from build123d import *
from build123d.topology import SkipClean

# Parameters (mm, degrees)
SKETCH_1_R              = 2.5
SKETCH_1_W              = 47.2
SKETCH_1_H              = 66.2
SKETCH_1_R_2            = 1.5
SKETCH_1_W_2            = 89
SKETCH_1_H_2            = 34
EXTRUDE_1_DEPTH         = 10
FILLET_1_R              = 4
FILLET_4_R              = 6
FILLET_7_R              = 3
FILLET_8_R              = 3
SKETCH_2_R              = 2.5
SKETCH_2_R_2            = 1.5
CUT_EXTRUDE_1_DEPTH     = 258.430709124
SKETCH_3_R              = 2.5
CUT_EXTRUDE_2_DEPTH     = 30
SKETCH_4_R              = 1.5
CUT_EXTRUDE_3_DEPTH     = 263.774751451
FILLET_10_R             = 15
FILLET_11_R             = 3
FILLET_1_OF_MIRROR_1_R  = 4
FILLET_4_OF_MIRROR_1_R  = 6
FILLET_7_OF_MIRROR_1_R  = 3
FILLET_8_OF_MIRROR_1_R  = 3
FILLET_10_OF_MIRROR_1_R = 15
FILLET_11_OF_MIRROR_1_R = 3
SKETCH_5_R              = 2.5
EXTRUDE_2_DEPTH         = 10
SKETCH_6_R              = 2.5
CUT_EXTRUDE_4_DEPTH     = 10
EXTRUDE_3_DEPTH         = 10
SKETCH_8_R              = 2.5
CUT_EXTRUDE_5_DEPTH     = 10


with BuildPart() as part:
    # 草图1 → 凸台-拉伸1 (new body)
    with BuildSketch(Plane.XY):
        with BuildLine():
            Line((-46, -17), (-46, 17))
            Line((-46, 17), (0, 17))
            Line((0, 17), (0, 25))
            Line((0, 25), (-176.776511015, 25))
            ThreePointArc((-176.776511015, 25), (-184.605554742, 35.220778596), (-194.787701414, 43.1))
            Line((-194.787701414, 43.1), (-203.153806011, 41.1))
            Line((-203.153806011, 41.1), (-236.846193989, 41.1))
            Line((-236.846193989, 41.1), (-245.212298586, 43.1))
            ThreePointArc((-245.212298586, 43.1), (-249.567187761, 40.23743789), (-253.6, 36.936567247))
            Line((-253.6, 36.936567247), (-253.6, 25.2))
            ThreePointArc((-253.6, 25.2), (-252.623320065, 26.452201949), (-251.6, 27.666586345))
            Line((-251.6, 27.666586345), (-251.6, -27.666586345))
            ThreePointArc((-251.6, -27.666586345), (-252.623320065, -26.452201949), (-253.6, -25.2))
            Line((-253.6, -25.2), (-253.6, -36.936567247))
            ThreePointArc((-253.6, -36.936567247), (-249.567187761, -40.23743789), (-245.212298586, -43.1))
            Line((-245.212298586, -43.1), (-236.846193989, -41.1))
            Line((-236.846193989, -41.1), (-203.153806011, -41.1))
            Line((-203.153806011, -41.1), (-194.787701414, -43.1))
            ThreePointArc((-194.787701414, -43.1), (-184.605554742, -35.220778596), (-176.776511015, -25))
            Line((-176.776511015, -25), (0, -25))
            Line((0, -25), (0, -17))
            Line((0, -17), (-46, -17))
        make_face()
        with Locations((-51, 17)):
            Circle(SKETCH_1_R, mode=Mode.SUBTRACT)
        with Locations((-150, -19)):
            Circle(SKETCH_1_R, mode=Mode.SUBTRACT)
        with BuildLine():
            Line((-188.4, -27.666586345), (-188.4, 27.666586345))
            ThreePointArc((-188.4, 27.666586345), (-178, 0), (-188.4, -27.666586345))
        make_face(mode=Mode.SUBTRACT)
        with BuildLine():
            Line((-155, -17), (-173.050346114, -17))
            ThreePointArc((-173.050346114, -17), (-170.067345354, 0), (-173.050346114, 17))
            Line((-173.050346114, 17), (-155, 17))
            Line((-155, 17), (-155, -17))
        make_face(mode=Mode.SUBTRACT)
        with Locations((-51, -17)):
            Circle(SKETCH_1_R, mode=Mode.SUBTRACT)
        with Locations((-220, 0)):
            Rectangle(SKETCH_1_W, SKETCH_1_H, mode=Mode.SUBTRACT)
        with Locations((-150, 0)):
            Circle(SKETCH_1_R_2, mode=Mode.SUBTRACT)
        with Locations((-150, 19)):
            Circle(SKETCH_1_R, mode=Mode.SUBTRACT)
        with Locations((-100.5, 0)):
            Rectangle(SKETCH_1_W_2, SKETCH_1_H_2, mode=Mode.SUBTRACT)
        with Locations((-51, 0)):
            Circle(SKETCH_1_R_2, mode=Mode.SUBTRACT)
    extrude_1 = extrude(amount=EXTRUDE_1_DEPTH)

    # 圆角1
    fillet_1_edges = [part.edges().sort_by_distance(p)[0] for p in [
        (-196.4, 33.1, 5),
        (-243.6, 33.1, 5),
        (-243.6, -33.1, 5),
        (-196.4, -33.1, 5),
    ]]
    fillet(fillet_1_edges, radius=FILLET_1_R)

    # 圆角4
    fillet_4_edges = [part.edges().sort_by_distance(p)[0] for p in [
        (-155, -17, 5),
        (-155, 17, 5),
        (-145, 17, 5),
        (-145, -17, 5),
        (-56, -17, 5),
        (-56, 17, 5),
        (-46, -17, 5),
        (-46, 17, 5),
    ]]
    fillet(fillet_4_edges, radius=FILLET_4_R)

    # 圆角7
    # the kernel refuses this fillet: 3 mm, written as the material it adds along each edge
    with BuildSketch(Plane(origin=(-251.6, -27.666586345, 0), x_dir=(-0.6298143321188929, 0.7767457158283095, 0), z_dir=(0, 0, 1))) as fillet_7_piece_1:
        with BuildLine():
            CenterArc((6.002322024, -1.004638225), FILLET_7_R, 160.43479501, 70.528779366)
            Line((4.112879028, -3.334875372), (4.075090168, -3.381480115))
            Line((4.075090168, -3.381480115), (-0.03778886, -0.046604743))
            Line((-0.03778886, -0.046604743), (-0.002268242, 0.05995711))
            ThreePointArc((-0.002268242, 0.05995711), (1.58776952, 0.090022779), (3.119003381, 0.020092764))
            Line((3.119003381, 0.020092764), (3.175539041, 0))
        make_face()
    extrude(amount=10)
    with BuildSketch(Plane(origin=(-251.6, 27.666586345, 0), x_dir=(0, -1, 0), z_dir=(0, 0, 1))) as fillet_7_piece_2:
        with BuildLine():
            CenterArc((5.29501347, -3), FILLET_7_R, 90, 70.528779366)
            Line((2.466586345, -2), (2.410017803, -1.98))
            ThreePointArc((2.410017803, -1.98), (1.176595536, -1.069924808), (-0.039523695, -0.045142857))
            Line((-0.039523695, -0.045142857), (0, 0.06))
            Line((0, 0.06), (5.29501347, 0.06))
            Line((5.29501347, 0.06), (5.29501347, 0))
        make_face()
    extrude(amount=10)

    # 圆角8
    fillet_8_edges = [part.edges().sort_by_distance(p)[0] for p in [
        (-188.4, 27.666586345, 5),
        (-188.4, -27.666586345, 5),
    ]]
    fillet(fillet_8_edges, radius=FILLET_8_R)

    # 草图2 → 切除-拉伸1 (cut, symmetric)
    with BuildSketch(Plane(origin=(0, 0, 0), x_dir=(1, 0, 0), z_dir=(0, 1, 0))):
        with Locations(Location((-232.5, -5, 0), (0, 0, 270))):
            Circle(SKETCH_2_R)
        with Locations(Location((-207.5, -5, 0), (0, 0, 270))):
            Circle(SKETCH_2_R)
        with Locations(Location((-220, -5, 0), (0, 0, 270))):
            Circle(SKETCH_2_R_2)
    cut_extrude_1 = extrude(amount=CUT_EXTRUDE_1_DEPTH, both=True, mode=Mode.SUBTRACT)

    # 草图3 → 切除-拉伸2 (cut)
    with BuildSketch(Plane(origin=(-243.6, 0, 0), x_dir=(0, 0, -1), z_dir=(1, 0, 0))):
        with Locations((-5, 15)):
            Circle(SKETCH_3_R)
        with Locations((-5, -15)):
            Circle(SKETCH_3_R)
    cut_extrude_2 = extrude(amount=-CUT_EXTRUDE_2_DEPTH, mode=Mode.SUBTRACT)

    # 草图4 → 切除-拉伸3 (cut, through all)
    with BuildSketch(Plane(origin=(0, 25, 0), x_dir=(1, 0, 0), z_dir=(0, 1, 0))):
        with Locations((0, -5)):
            Circle(SKETCH_4_R)
    cut_extrude_3 = extrude(amount=-CUT_EXTRUDE_3_DEPTH, mode=Mode.SUBTRACT)

    # 圆角10
    fillet_10_edges = [part.edges().sort_by_distance(p)[0] for p in [
        (-176.776511015, -25, 5),
        (-176.776511015, 25, 5),
    ]]
    fillet(fillet_10_edges, radius=FILLET_10_R)

    # 圆角11
    fillet_11_edges = [part.edges().sort_by_distance(p)[0] for p in [
        (-173.050346114, 17, 5),
        (-173.050346114, -17, 5),
    ]]
    fillet(fillet_11_edges, radius=FILLET_11_R)

    # 镜向1: 凸台-拉伸1, 切除-拉伸1, 切除-拉伸2, 切除-拉伸3 across plane
    with SkipClean():  # the faces are left unmerged after this step: merging them gives an invalid solid
        add(extrude_1.mirror(Plane(origin=(0, 0, 10), x_dir=(0, 0, 1), z_dir=(1, 0, 0))))
        add(cut_extrude_1.mirror(Plane(origin=(0, 0, 10), x_dir=(0, 0, 1), z_dir=(1, 0, 0))), mode=Mode.SUBTRACT)
        add(cut_extrude_2.mirror(Plane(origin=(0, 0, 10), x_dir=(0, 0, 1), z_dir=(1, 0, 0))), mode=Mode.SUBTRACT)
        add(cut_extrude_3.mirror(Plane(origin=(0, 0, 10), x_dir=(0, 0, 1), z_dir=(1, 0, 0))), mode=Mode.SUBTRACT)

    # 圆角1 of 镜向1
    fillet_1_of_mirror_1_edges = [part.edges().sort_by_distance(p)[0] for p in [
        (196.4, 33.1, 5),
        (243.6, 33.1, 5),
        (243.6, -33.1, 5),
        (196.4, -33.1, 5),
    ]]
    fillet(fillet_1_of_mirror_1_edges, radius=FILLET_1_OF_MIRROR_1_R)

    # 圆角4 of 镜向1
    fillet_4_of_mirror_1_edges = [part.edges().sort_by_distance(p)[0] for p in [
        (155, -17, 5),
        (155, 17, 5),
        (145, 17, 5),
        (145, -17, 5),
        (56, -17, 5),
        (56, 17, 5),
        (46, -17, 5),
        (46, 17, 5),
    ]]
    fillet(fillet_4_of_mirror_1_edges, radius=FILLET_4_OF_MIRROR_1_R)

    # 圆角7 of 镜向1
    # the kernel refuses this fillet: 3 mm, written as the material it adds along each edge
    with BuildSketch(Plane(origin=(251.6, -27.666586345, 0), x_dir=(0, 1, 0), z_dir=(0, 0, 1))) as fillet_7_of_mirror_1_piece_1:
        with BuildLine():
            CenterArc((5.29501347, -3), FILLET_7_OF_MIRROR_1_R, 90, 70.528779366)
            Line((2.466586345, -2), (2.410017803, -1.98))
            ThreePointArc((2.410017803, -1.98), (1.176595536, -1.069924808), (-0.039523695, -0.045142857))
            Line((-0.039523695, -0.045142857), (0, 0.06))
            Line((0, 0.06), (5.29501347, 0.06))
            Line((5.29501347, 0.06), (5.29501347, 0))
        make_face()
    extrude(amount=10)
    with BuildSketch(Plane(origin=(251.6, 27.666586345, 0), x_dir=(0.6298143321188939, -0.7767457158283085, 0), z_dir=(0, 0, 1))) as fillet_7_of_mirror_1_piece_2:
        with BuildLine():
            CenterArc((6.002322024, -1.004638225), FILLET_7_OF_MIRROR_1_R, 160.43479501, 70.528779366)
            Line((4.112879028, -3.334875372), (4.075090168, -3.381480115))
            Line((4.075090168, -3.381480115), (-0.03778886, -0.046604743))
            Line((-0.03778886, -0.046604743), (-0.002268242, 0.05995711))
            ThreePointArc((-0.002268242, 0.05995711), (1.58776952, 0.090022779), (3.119003381, 0.020092764))
            Line((3.119003381, 0.020092764), (3.175539041, 0))
        make_face()
    extrude(amount=10)

    # 圆角8 of 镜向1
    fillet_8_of_mirror_1_edges = [part.edges().sort_by_distance(p)[0] for p in [
        (188.4, 27.666586345, 5),
        (188.4, -27.666586345, 5),
    ]]
    fillet(fillet_8_of_mirror_1_edges, radius=FILLET_8_OF_MIRROR_1_R)

    # 圆角10 of 镜向1
    fillet_10_of_mirror_1_edges = [part.edges().sort_by_distance(p)[0] for p in [
        (176.776511015, -25, 5),
        (176.776511015, 25, 5),
    ]]
    fillet(fillet_10_of_mirror_1_edges, radius=FILLET_10_OF_MIRROR_1_R)

    # 圆角11 of 镜向1
    fillet_11_of_mirror_1_edges = [part.edges().sort_by_distance(p)[0] for p in [
        (173.050346114, 17, 5),
        (173.050346114, -17, 5),
    ]]
    fillet(fillet_11_of_mirror_1_edges, radius=FILLET_11_OF_MIRROR_1_R)

    # 草图5 → 凸台-拉伸2 (add)
    with BuildSketch(Plane(origin=(0, 0, 0), x_dir=(-1, 0, 0), z_dir=(0, 0, -1))):
        with Locations((150, 19)):
            Circle(SKETCH_5_R)
        with Locations((150, -19)):
            Circle(SKETCH_5_R)
        with Locations((-150, -19)):
            Circle(SKETCH_5_R)
        with Locations((-150, 19)):
            Circle(SKETCH_5_R)
    extrude(amount=-EXTRUDE_2_DEPTH)

    # 草图6 → 切除-拉伸4 (cut)
    with BuildSketch(Plane(origin=(0, 0, 0), x_dir=(-1, 0, 0), z_dir=(0, 0, -1))):
        with Locations(Location((-150, 16, 0), (0, 0, 90))):
            Circle(SKETCH_6_R)
        with Locations(Location((-150, -16, 0), (0, 0, 270))):
            Circle(SKETCH_6_R)
        with Locations((48, -16)):
            Circle(SKETCH_6_R)
        with Locations((48, 16)):
            Circle(SKETCH_6_R)
    extrude(amount=-CUT_EXTRUDE_4_DEPTH, mode=Mode.SUBTRACT)

    # 草图7 → 凸台-拉伸3 (add)
    with BuildSketch(Plane(origin=(0, 0, 0), x_dir=(-1, 0, 0), z_dir=(0, 0, -1))):
        with BuildLine():
            ThreePointArc((48.887627564, 18.337117307), (45.628291755, 15.209430585), (50.112372436, 14.662882693))
            ThreePointArc((50.112372436, 14.662882693), (48.628291755, 16.209430585), (48.887627564, 18.337117307))
        make_face()
        with BuildLine():
            ThreePointArc((50.112372436, -14.662882693), (48.628291755, -16.209430585), (48.887627564, -18.337117307))
            ThreePointArc((48.887627564, -18.337117307), (45.628291755, -15.209430585), (50.112372436, -14.662882693))
        make_face()
    extrude(amount=-EXTRUDE_3_DEPTH)

    # 草图8 → 切除-拉伸5 (cut)
    with BuildSketch(Plane(origin=(0, 0, 0), x_dir=(-1, 0, 0), z_dir=(0, 0, -1))):
        with Locations(Location((-150, 16, 0), (0, 0, 90))):
            Circle(SKETCH_8_R)
        with Locations(Location((-150, -16, 0), (0, 0, 270))):
            Circle(SKETCH_8_R)
        with Locations(Location((150, -16, 0), (0, 0, 270))):
            Circle(SKETCH_8_R)
        with Locations(Location((150, 16, 0), (0, 0, 270))):
            Circle(SKETCH_8_R)
    extrude(amount=-CUT_EXTRUDE_5_DEPTH, mode=Mode.SUBTRACT)


solid = part.part
Model file for the job. Use its own axes, mm. A direction names the side the tool comes from. Give positions to 0.01 mm unless a question says otherwise; leave off trailing zeros. Loops run counter-clockwise (first coordinate to the right, second up) from the corner with the lowest first, then second, coordinate; pieces in that order, holes last. Notation, with made-up numbers: (63, 57) -> (67, 57) arc R22 cw to (67, 91) -> close; hole circle Ø2 at (-31, -2.75). An arc over 180 degrees is marked (long way). Use a Markdown table: item, result. Add a question column.
(1) Tool access for faces 1 (the flat face through (220, 41.1, 3)), 2 (the cylindrical face through (-187.242, -37.685, 4.93)), 3 (the flat face through (56, 0, 5)): list every direction of +Z, -Z, +X, -X, +Y, -Y with a clear straight run to the whole face (end or side of a thin tool).
(2) Drop flat-ended pins along their axis: pin 1 Ø5 at (x, z) = (11, 5) entering from +Y; pin 2 Ø3 at (x, z) = (216, 4.5) entering from +Y; pin 3 Ø3 at (x, z) = (220.5, 7.5) entering from -Y; pin 4 Ø12 at (x, y) = (-39, -34) entering from +Z. Give the stop position or say it passes through.
(3) Slice it at A-A on x = -98.5. List the corners of the cut face in (y, z), and give its area (3 significant figures).
(4) Wall check: line 1 along Y through (x, z) = (96.5, 8); line 2 along Y through (x, z) = (51, 3); line 3 along Y through (x, z) = (-150, 7). Give the ranges that are in metal, low to high.
(5) Mould opens along Y. For faces 4 (the flat face through (-165, -17, 5)), 5 (the cylindrical face through (249.51, 40.28, 4.93)), 6 (the flat face through (-220, 33.1, 3)), 7 (the flat face through (2, -25, 5)) say: +Y half, -Y half, draft (parallel to the pull), parting line (faces both ways), or undercut.
Filled sheet:
| question | item | result |
|---|---|---|
| 1 | face 1 | +Z, -Z, +Y |
| 1 | face 2 | +Z, -Z, -Y |
| 1 | face 3 | +Z, -Z |
| 2 | pin 1 | y = 25 |
| 2 | pin 2 | y = 41.1 |
| 2 | pin 3 | y = -41.1 |
| 2 | pin 4 | through |
| 3 | outline | (-25, 0) -> (-17, 0) -> (-17, 10) -> (-25, 10) -> close; (17, 0) -> (25, 0) -> (25, 10) -> (17, 10) -> close |
| 3 | area | 160 mm2 |
| 4 | line 1 | -25 to -17, 17 to 25 |
| 4 | line 2 | -25 to -19.5, -14.5 to -1.5, 1.5 to 14.5, 19.5 to 25 |
| 4 | line 3 | -25 to -18.5, -13.5 to -1.5, 1.5 to 13.5, 18.5 to 25 |
| 5 | face 4 | undercut |
| 5 | face 5 | +Y half |
| 5 | face 6 | undercut |
| 5 | face 7 | -Y half |
